The model under review builds one solid part; all positions refer to its coordinate system, in mm. A direction names the side the tool comes from. Give positions to 0.01 mm unless a question says otherwise; leave off trailing zeros.
```python
from build123d import *

# Parameters (mm, degrees)
BOX009_W     = 275
BOX009_H     = 275
BOX009_DEPTH = 59
SKETCH036_W  = 101
SKETCH036_H  = 101
SKETCH037_W  = 85
SKETCH037_H  = 85
BOX008_W     = 275
BOX008_H     = 275
BOX008_DEPTH = 52
SKETCH034_W  = 275
SKETCH034_H  = 275
SKETCH035_W  = 0.1
SKETCH035_H  = 0.1
BOX007_W     = 275
BOX007_H     = 275
BOX007_DEPTH = 47
SKETCH032_W  = 195
SKETCH032_H  = 195
SKETCH033_W  = 180
SKETCH033_H  = 180
BOX006_W     = 275
BOX006_H     = 275
BOX006_DEPTH = 52
SKETCH030_W  = 275
SKETCH030_H  = 275
SKETCH031_W  = 0.1
SKETCH031_H  = 0.1
SKETCH028_W  = 275
SKETCH028_H  = 275
SKETCH029_W  = 0.1
SKETCH029_H  = 0.1
BOX005_W     = 275
BOX005_H     = 275
BOX005_DEPTH = 57
BOX004_W     = 275
BOX004_H     = 275
BOX004_DEPTH = 55
SKETCH026_W  = 275
SKETCH026_H  = 275
SKETCH027_W  = 0.1
SKETCH027_H  = 0.1
SKETCH024_W  = 275
SKETCH024_H  = 275
SKETCH025_W  = 0.1
SKETCH025_H  = 0.1
BOX003_W     = 275
BOX003_H     = 275
BOX003_DEPTH = 70


with BuildPart() as layer0keep004:
    # Box009 → Box009 (new body)
    with BuildSketch(Plane.XY.offset(48)):
        with Locations((137.5, 137.5)):
            Rectangle(BOX009_W, BOX009_H)
    extrude(amount=BOX009_DEPTH)


with BuildPart() as obj1:
    # Sketch036 → Loft010 section 0
    with BuildSketch(Plane.XY.offset(107)):
        with Locations((137.5, 137.5)):
            Rectangle(SKETCH036_W, SKETCH036_H)
    # Sketch037 → Loft010 section 1
    with BuildSketch(Plane.XY.offset(117)):
        with Locations((137.5, 137.5)):
            Rectangle(SKETCH037_W, SKETCH037_H)
    loft()

    # Fusion018: union layer0Keep004
    add(layer0keep004.part)


with BuildPart() as layer013:
    # Box008 → Box008 (new body)
    with BuildSketch(Plane.XY.offset(5)):
        with Locations((137.5, 137.5)):
            Rectangle(BOX008_W, BOX008_H)
    extrude(amount=BOX008_DEPTH)


with BuildPart() as obj2:
    # Sketch034 → Loft009 section 0
    with BuildSketch(Plane.XY):
        with Locations((137.5, 137.5)):
            Rectangle(SKETCH034_W, SKETCH034_H)
    # Sketch035 → Loft009 section 1
    with BuildSketch(Plane.XY.offset(175.1)):
        with Locations((137.5, 137.5)):
            Rectangle(SKETCH035_W, SKETCH035_H)
    loft()


with BuildPart() as obj2_1:
    # Loft009 placement: moved
    add(obj2.part.moved(Location((0, 0, -6))))

    # Common008: intersect layer013
    add(layer013.part, mode=Mode.INTERSECT)


with BuildPart() as layer0keep002:
    # Box007 → Box007 (new body)
    with BuildSketch(Plane.XY):
        with Locations((137.5, 137.5)):
            Rectangle(BOX007_W, BOX007_H)
    extrude(amount=BOX007_DEPTH)


with BuildPart() as layer012:
    # Sketch032 → Loft008 section 0
    with BuildSketch(Plane.XY.offset(47)):
        with Locations((137.5, 137.5)):
            Rectangle(SKETCH032_W, SKETCH032_H)
    # Sketch033 → Loft008 section 1
    with BuildSketch(Plane.XY.offset(57)):
        with Locations((137.5, 137.5)):
            Rectangle(SKETCH033_W, SKETCH033_H)
    loft()

    # Fusion016: union layer0Keep002
    add(layer0keep002.part)


with BuildPart() as layer009:
    # Box006 → Box006 (new body)
    with BuildSketch(Plane.XY.offset(5)):
        with Locations((137.5, 137.5)):
            Rectangle(BOX006_W, BOX006_H)
    extrude(amount=BOX006_DEPTH)


with BuildPart() as layer0cut002:
    # Sketch030 → Loft007 section 0
    with BuildSketch(Plane.XY):
        with Locations((137.5, 137.5)):
            Rectangle(SKETCH030_W, SKETCH030_H)
    # Sketch031 → Loft007 section 1
    with BuildSketch(Plane.XY.offset(175.1)):
        with Locations((137.5, 137.5)):
            Rectangle(SKETCH031_W, SKETCH031_H)
    loft()


with BuildPart() as layer0cut002_1:
    # Loft007 placement: moved
    add(layer0cut002.part.moved(Location((0, 0, -6))))

    # Common006: intersect layer009
    add(layer009.part, mode=Mode.INTERSECT)


with BuildPart() as obj3:
    # Sketch028 → Loft006 section 0
    with BuildSketch(Plane.XY):
        with Locations((137.5, 137.5)):
            Rectangle(SKETCH028_W, SKETCH028_H)
    # Sketch029 → Loft006 section 1
    with BuildSketch(Plane.XY.offset(175.1)):
        with Locations((137.5, 137.5)):
            Rectangle(SKETCH029_W, SKETCH029_H)
    loft()


with BuildPart() as obj4:
    # Box005 → Box005 (new body)
    with BuildSketch(Plane.XY):
        with Locations((137.5, 137.5)):
            Rectangle(BOX005_W, BOX005_H)
    extrude(amount=BOX005_DEPTH)

    # Common005: intersect obj3
    add(obj3.part, mode=Mode.INTERSECT)

    # Cut002: cut layer0cut002
    add(layer0cut002_1.part, mode=Mode.SUBTRACT)

    # Common007: intersect layer012
    add(layer012.part, mode=Mode.INTERSECT)

    # Fusion017: union obj2
    add(obj2_1.part)


with BuildPart() as obj4_1:
    # Fusion017 placement: moved
    add(obj4.part.moved(Location((0, 0, 1))))


with BuildPart() as layer005:
    # Box004 → Box004 (new body)
    with BuildSketch(Plane.XY.offset(62)):
        with Locations((137.5, 137.5)):
            Rectangle(BOX004_W, BOX004_H)
    extrude(amount=BOX004_DEPTH)


with BuildPart() as layer0cut001:
    # Sketch026 → Loft005 section 0
    with BuildSketch(Plane.XY):
        with Locations((137.5, 137.5)):
            Rectangle(SKETCH026_W, SKETCH026_H)
    # Sketch027 → Loft005 section 1
    with BuildSketch(Plane.XY.offset(175.1)):
        with Locations((137.5, 137.5)):
            Rectangle(SKETCH027_W, SKETCH027_H)
    loft()


with BuildPart() as layer0cut001_1:
    # Loft005 placement: moved
    add(layer0cut001.part.moved(Location((0, 0, -6))))

    # Common004: intersect layer005
    add(layer005.part, mode=Mode.INTERSECT)


with BuildPart() as obj5:
    # Sketch024 → Loft004 section 0
    with BuildSketch(Plane.XY):
        with Locations((137.5, 137.5)):
            Rectangle(SKETCH024_W, SKETCH024_H)
    # Sketch025 → Loft004 section 1
    with BuildSketch(Plane.XY.offset(175.1)):
        with Locations((137.5, 137.5)):
            Rectangle(SKETCH025_W, SKETCH025_H)
    loft()


with BuildPart() as obj6:
    # Box003 → Box003 (new body)
    with BuildSketch(Plane.XY.offset(47)):
        with Locations((137.5, 137.5)):
            Rectangle(BOX003_W, BOX003_H)
    extrude(amount=BOX003_DEPTH)

    # Common003: intersect obj5
    add(obj5.part, mode=Mode.INTERSECT)

    # Cut001: cut layer0cut001
    add(layer0cut001_1.part, mode=Mode.SUBTRACT)

    # Cut003: cut obj4
    add(obj4_1.part, mode=Mode.SUBTRACT)

    # Common009: intersect obj1
    add(obj1.part, mode=Mode.INTERSECT)


solid = obj6.part
```
Item 1: Draft analysis for pull direction Y (two halves, no side actions). For faces 3 (the flat face through (133, 86, 107)), 4 (the flat face through (136, 139, 62)), state which applies: released by +Y, released by -Y, zero draft, split by the parting line, or undercut.
Values found:
face 3: zero draft
face 4: undercut
Item 2: Clearance check with flat-ended pins moving along their axes: pin 1 Ø8 at (x, y) = (154, 193) entering from -Z; pin 2 Ø10 at (x, z) = (140.5, 100) entering from +Y; pin 3 Ø5 at (y, z) = (71.5, 70.5) entering from +X. State where each tip first meets the part, or that it passes through.
Values found:
pin 1: stops at z = 58
pin 2: stops at y = 200.43
pin 3: stops at x = 221.62
Item 3: For line 1 (Z direction, x = 120.5, y = 141.5); line 2 (X direction, y = 149, z = 110); line 3 (Y direction, x = 177, z = 53.5) (3 decimals), list the stretches that pass through material, from the lowest coordinate up.
Values found:
line 1: z = 58 to 62
line 2: x = 89.4 to 91.06, 183.94 to 185.6
line 3: y = 41.996 to 44.125, 230.875 to 233.004
Item 4: For faces 1 (the flat face through (136, 139, 58)), 2 (the flat face through (96, 157, 117)), list the 3-axis set-ups (+Z, -Z, +X, -X, +Y, -Y) from which the entire face can be reached by the end or side of a thin tool; tool diameter is ignored.
Values found:
face 1: -Z
face 2: +Z, +X, -X, +Y, -Y
